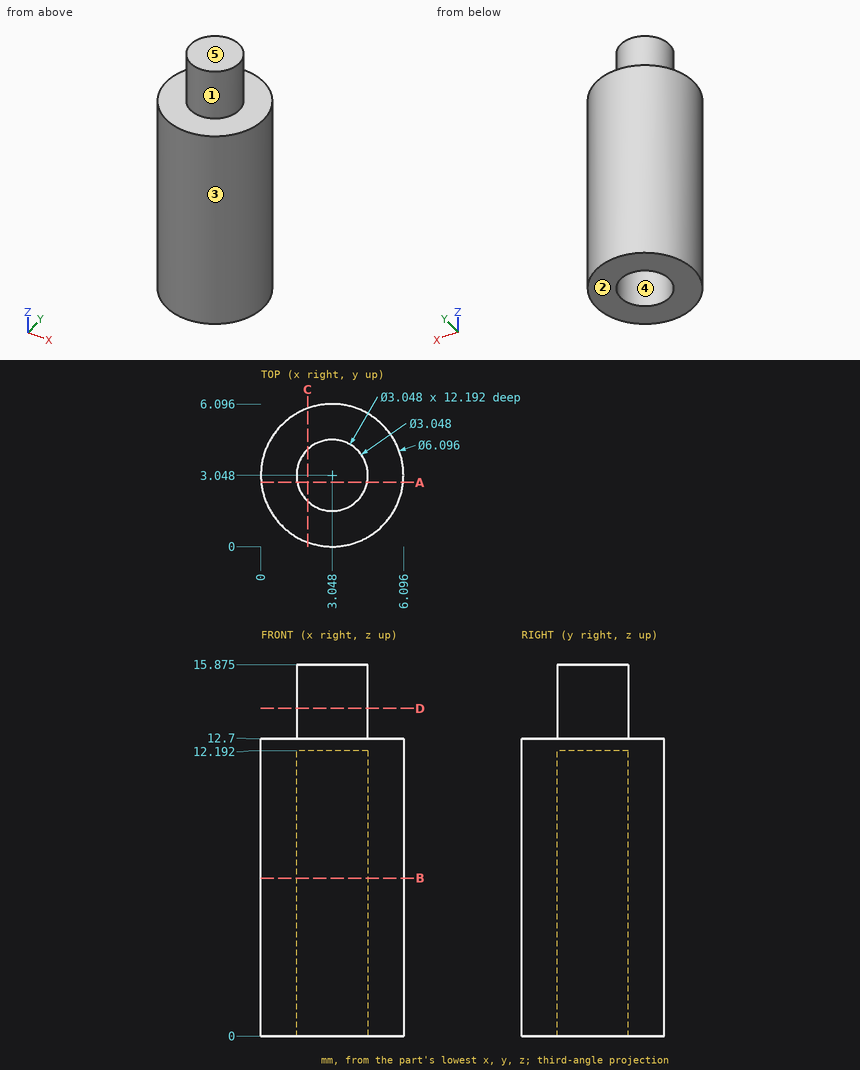
Print and shaded views of the part. All mm, measured from the part's lowest x, y and z. A direction names the side the tool comes from. Coordinates: 2 decimals unless noted, no trailing zeros. Loops run counter-clockwise (first coordinate to the right, second up) from the corner with the lowest first, then second, coordinate; pieces in that order, holes last. Notation, with made-up numbers: (-20.5, -11) - (22.5, -11) arc R28 ccw to (22.5, 18) - close; hole circle Ø1 at (-35.75, 35). An arc over 180 degrees is marked (long way). Write item = value, one per line. Start each with the question number.
Item 1: Saw through at D-D, the plane z = 14. List the corners of the cut face in (x, y), then the cut area to 3 significant figures.
Item 2: Wall check: probe 1 along X at (y, z) = (3, 9.5); probe 2 along Z at (x, y) = (2.75, 4) (3 decimals); probe 3 along Z at (x, y) = (3, 0.75). Give the ranges that are in metal, low to high. Write a range as [from, to].
Item 3: Pull direction Y, two halves, no side cores. Call the marked faces 3, 4 and 5: +Y half, -Y half, draft (parallel to the pull), parting line (faces both ways), or undercut.
Item 4: Saw through at A-A, the plane y = 2.75. List the corners of the cut face in (x, z) (3 decimals).
Item 5: Saw through at B-B, the plane z = 6.75. List the corners of the cut face in (x, y), then the cut area to 3 significant figures.
Item 6: Drop a flat-ended pin along its axis: pin 1 Ø1.5 at (y, z) = (4.5, 8.5) entering from -X. Give the stop position or say it passes through.
Item 7: Saw through at C-C, the plane x = 2. List the corners of the cut face in (y, z) (3 decimals).
Item 8: 3-axis set-ups, long thin cutter, end or side, ignore diameter. For the marked faces 1 and 2: which of +Z, -Z, +X, -X, +Y, -Y reach the whole face in a straight line?
Answers:
q1.outline = circle Ø3.05 at (3.05, 3.05)
q1.area = 7.30 mm2
q2.probe_1 = [0, 1.52], [4.57, 6.1]
q2.probe_2 = [12.192, 15.875]
q2.probe_3 = [0, 12.7]
q3.face_3 = parting line
q3.face_4 = undercut
q3.face_5 = draft
q4.outline = (0.015, 0) - (1.553, 0) - (1.553, 12.192) - (4.543, 12.192) - (4.543, 0) - (6.081, 0) - (6.081, 12.7) - (4.543, 12.7) - (4.543, 15.875) - (1.553, 15.875) - (1.553, 12.7) - (0.015, 12.7) - close
q5.outline = circle Ø6.1 at (3.05, 3.05); hole circle Ø3.05 at (3.05, 3.05)
q5.area = 21.9 mm2
q6.pin_1 = 0.08
q7.outline = (0.186, 0) - (1.942, 0) - (1.942, 12.192) - (4.154, 12.192) - (4.154, 0) - (5.91, 0) - (5.91, 12.7) - (4.154, 12.7) - (4.154, 15.875) - (1.942, 15.875) - (1.942, 12.7) - (0.186, 12.7) - close
q8.face_1 = +Z
q8.face_2 = -Z, +X, -X, +Y, -Y
